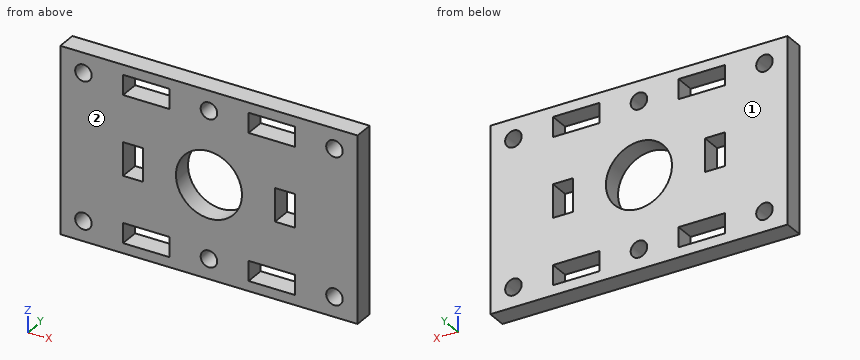
from build123d import *

# Parameters (mm, degrees)
SKETCH_1_W          = 45
SKETCH_1_H          = 28
EXTRUDE_1_DEPTH     = 3
SKETCH_2_R          = 1.25
SKETCH_2_W          = 7
SKETCH_2_H          = 3
CUT_EXTRUDE_1_DEPTH = 4
SKETCH_3_W          = 3
SKETCH_3_H          = 5
CUT_EXTRUDE_2_DEPTH = 4
SKETCH_4_R          = 5
CUT_EXTRUDE_3_DEPTH = 10


with BuildPart() as part:
    # 스케치1 → 보스-돌출1 (new body)
    with BuildSketch(Plane(origin=(0, 0, 0), x_dir=(1, 0, 0), z_dir=(0, 1, 0))):
        with Locations((22.5, 14)):
            Rectangle(SKETCH_1_W, SKETCH_1_H)
    extrude(amount=EXTRUDE_1_DEPTH)

    # 스케치2 → 컷-돌출1 (cut, through all)
    with BuildSketch(Plane(origin=(0, 3, 0), x_dir=(1, 0, 0), z_dir=(0, 1, 0))):
        with Locations((22.5, 3)):
            Circle(SKETCH_2_R)
        with Locations((22.5, 25)):
            Circle(SKETCH_2_R)
        with Locations((3.5, 3)):
            Circle(SKETCH_2_R)
        with Locations((41.5, 3)):
            Circle(SKETCH_2_R)
        with Locations((41.5, 25)):
            Circle(SKETCH_2_R)
        with Locations((3.5, 25)):
            Circle(SKETCH_2_R)
        with Locations((32, 3)):
            Rectangle(SKETCH_2_W, SKETCH_2_H)
        with Locations((13, 3)):
            Rectangle(SKETCH_2_W, SKETCH_2_H)
        with Locations((32, 25)):
            Rectangle(SKETCH_2_W, SKETCH_2_H)
        with Locations((13, 25)):
            Rectangle(SKETCH_2_W, SKETCH_2_H)
    extrude(amount=-CUT_EXTRUDE_1_DEPTH, mode=Mode.SUBTRACT)

    # 스케치3 → 컷-돌출2 (cut, through all)
    with BuildSketch(Plane(origin=(0, 3, 0), x_dir=(1, 0, 0), z_dir=(0, 1, 0))):
        with Locations((11, 14)):
            Rectangle(SKETCH_3_W, SKETCH_3_H)
        with Locations((34, 14)):
            Rectangle(SKETCH_3_W, SKETCH_3_H)
    extrude(amount=-CUT_EXTRUDE_2_DEPTH, mode=Mode.SUBTRACT)

    # 스케치4 → 컷-돌출3 (cut)
    with BuildSketch(Plane(origin=(0, 3, 0), x_dir=(1, 0, 0), z_dir=(0, 1, 0))):
        with Locations((22.5, 14)):
            Circle(SKETCH_4_R)
    extrude(amount=-CUT_EXTRUDE_3_DEPTH, mode=Mode.SUBTRACT)


solid = part.part
Can you work these out from the model? Positions are in its coordinate system, mm. Face numbers are marked on the shaded views. Give positions to 0.01 mm unless a question says otherwise; leave off trailing zeros. Order: outer loops, then holes, each group sorted by start corner. A loop starts at its lowest first (then second) coordinate and runs counter-clockwise, first axis right, second up. Notation, with made-up numbers: M 70.5,38.5 L 84.5,38.5 A14 cw 84.5,53.5 Z; hole C -39.5,47 d1. An arc over 180 degrees is marked long. Use a Markdown table: item, result. Add a question column.
Item 1: We'd pull the mould along Y, two halves only. Please class the marked faces 1 and 2: +Y half, -Y half, draft (parallel to the pull), parting line (faces both ways), or undercut.
Item 2: Suppose I cut it at D-D (z = -14). List the corners of the cut face in (x, y) for me.
Item 3: Suppose I cut it at B-B (z = -3). List the corners of the cut face in (x, y) for me.
Item 4: Suppose I cut it at C-C (x = 33.5). List the corners of the cut face in (y, z) for me, then the cut area to 3 significant figures.
Item 5: If I drill on L1, parallel to X at y = 2.3, z = -3; L2, parallel to Z at x = 3.5, y = 1.95; L3, parallel to Z at x = 22.5, y = 1.2, over which ranges is the centre line in solid material (lowest first)? Write a range as [from, to].
Item 6: Suppose I cut it at A-A (x = 3.5). List the corners of the cut face in (y, z) for me.
Answer sheet:
| question | item | result |
|---|---|---|
| 1 | face 1 | +Y half |
| 1 | face 2 | -Y half |
| 2 | outline | M 0,0 L 9.5,0 L 9.5,3 L 0,3 Z; M 12.5,0 L 17.5,0 L 17.5,3 L 12.5,3 Z; M 27.5,0 L 32.5,0 L 32.5,3 L 27.5,3 Z; M 35.5,0 L 45,0 L 45,3 L 35.5,3 Z |
| 3 | outline | M 0,0 L 2.25,0 L 2.25,3 L 0,3 Z; M 4.75,0 L 9.5,0 L 9.5,3 L 4.75,3 Z; M 16.5,0 L 21.25,0 L 21.25,3 L 16.5,3 Z; M 23.75,0 L 28.5,0 L 28.5,3 L 23.75,3 Z; M 35.5,0 L 40.25,0 L 40.25,3 L 35.5,3 Z; M 42.75,0 L 45,0 L 45,3 L 42.75,3 Z |
| 4 | outline | M 0,-28 L 3,-28 L 3,-26.5 L 0,-26.5 Z; M 0,-23.5 L 3,-23.5 L 3,-16.5 L 0,-16.5 Z; M 0,-11.5 L 3,-11.5 L 3,-4.5 L 0,-4.5 Z; M 0,-1.5 L 3,-1.5 L 3,0 L 0,0 Z |
| 4 | area | 51.0 mm² |
| 5 | L1 | x = [0, 2.25], [4.75, 9.5], [16.5, 21.25], [23.75, 28.5], [35.5, 40.25], [42.75, 45] |
| 5 | L2 | z = [-28, -26.25], [-23.75, -4.25], [-1.75, 0] |
| 5 | L3 | z = [-28, -26.25], [-23.75, -19], [-9, -4.25], [-1.75, 0] |
| 6 | outline | M 0,-28 L 3,-28 L 3,-26.25 L 0,-26.25 Z; M 0,-23.75 L 3,-23.75 L 3,-4.25 L 0,-4.25 Z; M 0,-1.75 L 3,-1.75 L 3,0 L 0,0 Z |
